Solid Edge part; units mm, degrees
sketch "Sketch1" plane through (0, 0, 0) normal (0, 0, 1) x (1, 0, 0)
  line L0 (-308, 10) -> (308, 10)
  line L1 (308, -10) -> (-308, -10)
  arc A0 (-308, -10) -> (-308, 10) centre (-308, 0) cw
  arc A1 (308, 10) -> (308, -10) centre (308, 0) cw
  circle A2 centre (-308, 0) radius 5
  circle A3 centre (308, 0) radius 5
  dimension "D1" = 308
  dimension "D2" = 308
extrude "Protrusion1" add sketch "Sketch1" against normal blind 5
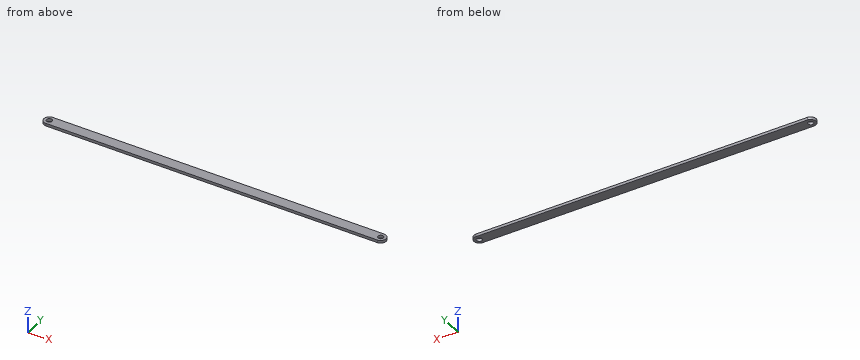
Source: CAD feature listing. Evaluate the final solid. Frame: model axes, mm. Round coordinates to 2 decimals unless told otherwise and drop trailing zeros. Loops run counter-clockwise (first coordinate to the right, second up) from the corner with the lowest first, then second, coordinate; pieces in that order, holes last.
Q1. First-contact query: P1, Ø3, axis at y = -6, z = -1, coming from the +X side; P2, Ø1, axis at y = -2.5, z = -1.5, coming from the -X side. Flat tips, straight axial feed; report the tip coordinate or a pass-through.
Q2. Ray query, line 1 (X direction, y = 1.5, z = -3.75); line 2 (X direction, y = -3, z = -3.5); line 3 (Y direction, x = -308, z = -2.1). Return the intervals inside material, ascending.
Q3. Section A-A, the plane z = -1.65. Return loops of the section in (x, y), plus the area to 3 significant figures.
Solutions:
1. P1: stops at x = 316.93
1. P2: stops at x = -317.8
2. line 1: x = -317.89 to -312.77, -303.23 to 303.23, 312.77 to 317.89
2. line 2: x = -317.54 to -312, -304 to 304, 312 to 317.54
2. line 3: y = -10 to -5, 5 to 10
3. outline: (-308, -10) - (308, -10) arc R10 ccw to (308, 10) - (-308, 10) arc R10 ccw to start; hole circle Ø10 at (-308, 0); hole circle Ø10 at (308, 0)
3. area: 12,500 mm2
